Design review of the part shown in the three views and the two pictorial views. Dimensions are in mm from the part's minimum x, y and z. Coordinates: 2 decimals unless noted, no trailing zeros. Loops run counter-clockwise (first coordinate to the right, second up) from the corner with the lowest first, then second, coordinate; pieces in that order, holes last. Notation, with made-up numbers: (-33.5, 21.5) -> (24.5, 21.5) arc R19 cw to (24.5, 26.5) -> close; hole circle Ø4 at (75.25, 37.5). An arc over 180 degrees is marked (long way). One line per item, written item: value.
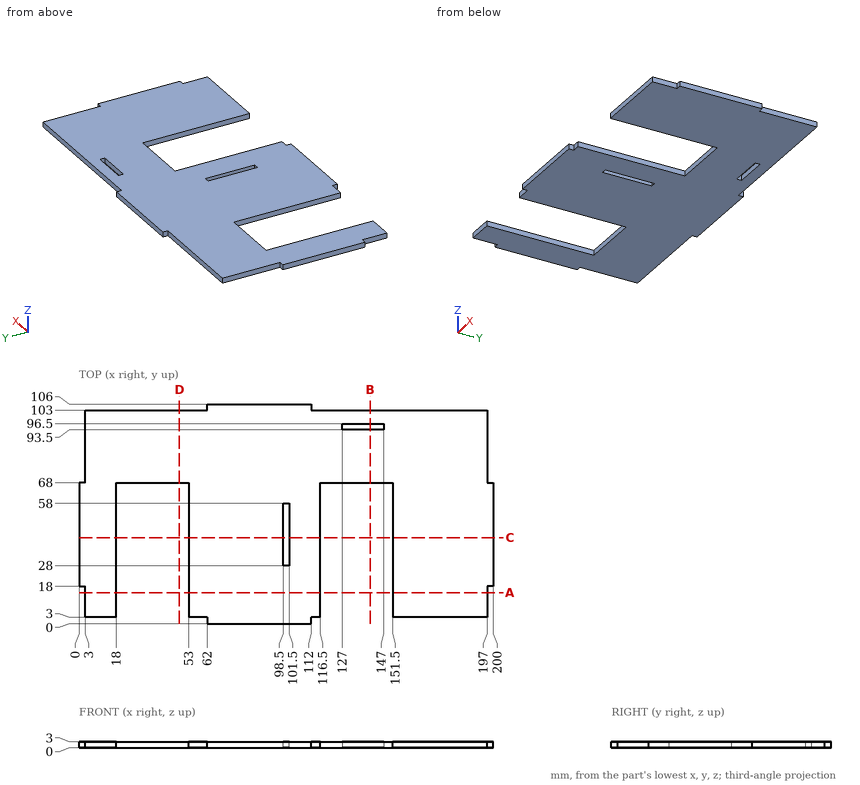
1. Take a section at A-A, the plane y = 15. Give the boundary of the cut face in (x, z).
Return value:
outline: (3, 0) -> (18, 0) -> (18, 3) -> (3, 3) -> close; (53, 0) -> (116.5, 0) -> (116.5, 3) -> (53, 3) -> close; (151.5, 0) -> (197, 0) -> (197, 3) -> (151.5, 3) -> close
2. To check wall thickness, follow probe 1 along X at (y, z) = (8, 1.3); probe 2 along X at (y, z) = (27, 2.2); probe 3 along X at (y, z) = (49.5, 0.7). State the ranges of each line that lie inside material, in increasing order. Write a range as from..to.
Return value:
probe 1: x = 3..18, 53..116.5, 151.5..197
probe 2: x = 0..18, 53..116.5, 151.5..200
probe 3: x = 0..18, 53..98.5, 101.5..116.5, 151.5..200
3. Take a section at D-D, the plane x = 48.5. Give the boundary of the cut face in (y, z), and give its area (3 significant figures).
Return value:
outline: (68, 0) -> (103, 0) -> (103, 3) -> (68, 3) -> close
area: 105 mm2
4. Take a section at C-C, the plane y = 41.5. Give the boundary of the cut face in (x, z), and give its area (3 significant figures).
Return value:
outline: (0, 0) -> (18, 0) -> (18, 3) -> (0, 3) -> close; (53, 0) -> (98.5, 0) -> (98.5, 3) -> (53, 3) -> close; (101.5, 0) -> (116.5, 0) -> (116.5, 3) -> (101.5, 3) -> close; (151.5, 0) -> (200, 0) -> (200, 3) -> (151.5, 3) -> close
area: 381 mm2
5. Take a section at B-B, the plane x = 140.5. Give the boundary of the cut face in (y, z), and give its area (3 significant figures).
Return value:
outline: (68, 0) -> (93.5, 0) -> (93.5, 3) -> (68, 3) -> close; (96.5, 0) -> (103, 0) -> (103, 3) -> (96.5, 3) -> close
area: 96.0 mm2
6. Insertion check: pin 1 Ø1.5 at (y, z) = (47.5, 0.5) entering from -X; pin 2 Ø1.5 at (x, z) = (2, 1) entering from -Y; pin 3 Ø1.5 at (x, z) = (113.5, 2) entering from -Y; pin 4 Ø1.5 at (y, z) = (9.5, 1) entering from +X. Each pin has a flat end and moves straight along its axis. Give the tip position at first contact, or say it passes through.
Return value:
pin 1: stops at x = 0
pin 2: stops at y = 18
pin 3: stops at y = 3
pin 4: stops at x = 197
